```python
from build123d import *

# Parameters (mm, degrees)
SKETCH1_W           = 107.95
SKETCH1_H           = 76.2
BOSS_EXTRUDE1_DEPTH = 31.75
SKETCH2_W           = 73.025
SKETCH2_H           = 5.715
CUT_EXTRUDE1_DEPTH  = 104.775
SKETCH3_R           = 1.8923
CUT_EXTRUDE2_DEPTH  = 32.75
SKETCH4_R           = 4.445
CUT_EXTRUDE3_DEPTH  = 2.54


with BuildPart() as part:
    # Sketch1 → Boss-Extrude1 (new body)
    with BuildSketch(Plane(origin=(0, 0, 0), x_dir=(1, 0, 0), z_dir=(0, 1, 0))):
        Rectangle(SKETCH1_W, SKETCH1_H)
    extrude(amount=BOSS_EXTRUDE1_DEPTH)

    # Sketch2 → Cut-Extrude1 (cut)
    with BuildSketch(Plane.ZY.offset(53.975)):
        with Locations((-1.5875, 25.7175)):
            Rectangle(SKETCH2_W, SKETCH2_H)
        with Locations((-1.5875, 18.520833333)):
            Rectangle(SKETCH2_W, SKETCH2_H)
        with Locations((-1.5875, 11.324166667)):
            Rectangle(SKETCH2_W, SKETCH2_H)
        with Locations((-1.5875, 4.1275)):
            Rectangle(SKETCH2_W, SKETCH2_H)
    extrude(amount=-CUT_EXTRUDE1_DEPTH, mode=Mode.SUBTRACT)

    # Sketch3 → Cut-Extrude2 (cut, through all)
    with BuildSketch(Plane(origin=(0, 31.75, 0), x_dir=(1, 0, 0), z_dir=(0, 1, 0))):
        with Locations((43.815, 29.21)):
            Circle(SKETCH3_R)
    extrude(amount=-CUT_EXTRUDE2_DEPTH, mode=Mode.SUBTRACT)

    # Sketch4 → Cut-Extrude3 (cut)
    with BuildSketch(Plane(origin=(0, 31.75, 0), x_dir=(1, 0, 0), z_dir=(0, 1, 0))):
        with Locations((43.815, 29.21)):
            Circle(SKETCH4_R)
    extrude(amount=-CUT_EXTRUDE3_DEPTH, mode=Mode.SUBTRACT)


solid = part.part
```
Model file for the job. Use its own axes, mm. A direction names the side the tool comes from. Round coordinates to 2 decimals unless told otherwise and drop trailing zeros. Write each loop counter-clockwise with the first axis right and the second up, starting at its lowest first coordinate (ties: lowest second). Pieces come first, ordered by that corner, then holes. Notation, with made-up numbers: M -5.75,81 L 29.25,81 A19 cw 29.25,90 Z; hole C 81,65 d1. An arc over 180 degrees is marked long. Put each result on its own line as item: value.
Item 1: Cut at D-D (z = -29.21). State how many separate pieces and enclosed holes the cut face has, and give its area (3 significant figures).
Responses:
separate pieces: 6
enclosed holes: 0
area: 986 mm²
Item 2: Mould opens along Z. For faces 1 (the cylindrical face through (48.055, 30.498, -30.545)), 2 (the flat face through (-53.975, 15, 3)), 3 (the flat face through (-2, 11, 34.925)) say: +Z half, -Z half, draft (parallel to the pull), parting line (faces both ways), or undercut.
Responses:
face 1: undercut
face 2: draft
face 3: -Z half
Item 3: Cut at C-C (x = 18). List the corners of the cut face in (y, z) (3 decimals), and give its area (3 significant figures).
Responses:
outline: M 0,-38.1 L 1.27,-38.1 L 1.27,34.925 L 6.985,34.925 L 6.985,-38.1 L 8.467,-38.1 L 8.467,34.925 L 14.182,34.925 L 14.182,-38.1 L 15.663,-38.1 L 15.663,34.925 L 21.378,34.925 L 21.378,-38.1 L 22.86,-38.1 L 22.86,34.925 L 28.575,34.925 L 28.575,-38.1 L 31.75,-38.1 L 31.75,38.1 L 0,38.1 Z
area: 750 mm²
Item 4: Tool access for faces 4 (the flat face through (-1, 31.75, -1)), 5 (the flat face through (44, 29.21, -27)), 6 (the flat face through (-2, 15.663, -2)): list every direction of +Z, -Z, +X, -X, +Y, -Y with a clear straight run to the whole face (end or side of a thin tool).
Responses:
face 4: +Z, -Z, +X, -X, +Y
face 5: +Y
face 6: -Z, -X
Item 5: Probe L1, parallel to Y at x = -26, z = -25 (3 decimals); L2, parallel to X at y = 15, z = -29 (3 decimals); L3, parallel to X at y = 11, z = -0.5 (3 decimals). List the from-to ranges inside material, lowest first. Write a range as from..to.
Responses:
L1: 0..1.27, 6.985..8.467, 14.182..15.663, 21.378..22.86, 28.575..31.75
L2: -53.975..41.934, 45.696..53.975
L3: 50.8..53.975
Item 6: Cut at B-B (y = 5). List the corners of the cut face in (x, z) (3 decimals).
Responses:
outline: M -53.975,34.925 L 50.8,34.925 L 50.8,-38.1 L 53.975,-38.1 L 53.975,38.1 L -53.975,38.1 Z
Item 7: Flat gauge pins, fed straight in: P1, Ø6.5, axis at x = -10.5, y = 26.5, coming from the -Z side; P2, Ø3, axis at y = 18.5, z = 16, coming from the -X side; P3, Ø1.7, axis at x = -24, y = 5.5, coming from the -Z side (3 decimals). Where does each tip first touch, or does it go through?
Responses:
P1: z = -38.1
P2: x = 50.8
P3: z = 34.925
Item 8: Cut at A-A (z = 5). List the corners of the cut face in (x, y) (3 decimals).
Responses:
outline: M -53.975,0 L 53.975,0 L 53.975,31.75 L -53.975,31.75 L -53.975,28.575 L 50.8,28.575 L 50.8,22.86 L -53.975,22.86 L -53.975,21.378 L 50.8,21.378 L 50.8,15.663 L -53.975,15.663 L -53.975,14.182 L 50.8,14.182 L 50.8,8.467 L -53.975,8.467 L -53.975,6.985 L 50.8,6.985 L 50.8,1.27 L -53.975,1.27 Z
